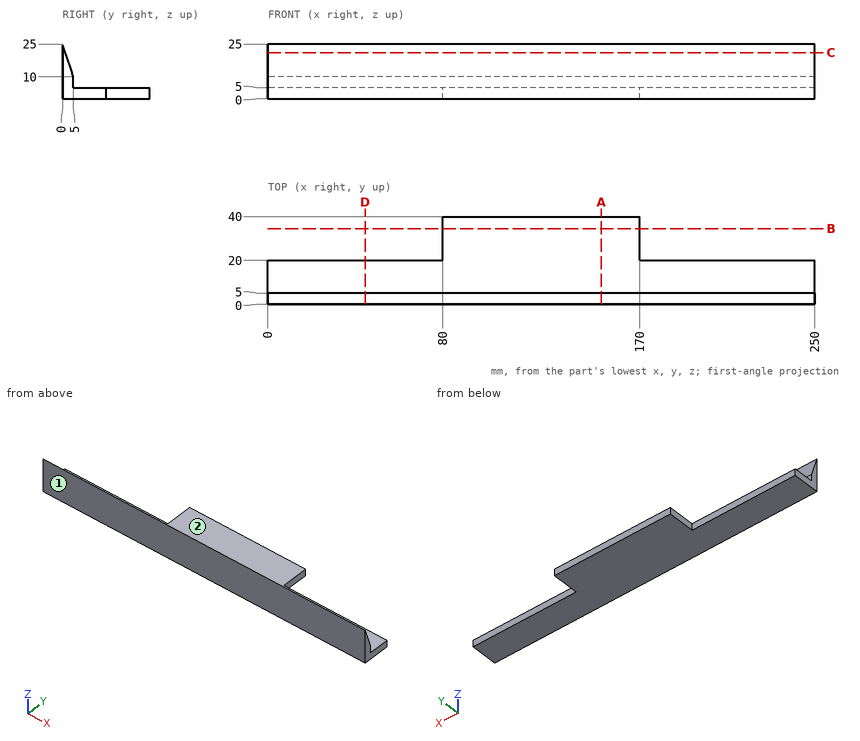
Answer from the drawing. Dimensions are ordinates in mm from the lowest x, y and z of the part. A direction names the side the tool comes from. Coordinates: 2 decimals unless noted, no trailing zeros. Write each loop counter-clockwise with the first axis right and the second up, starting at its lowest first coordinate (ties: lowest second). Pieces come first, ordered by that corner, then holes. Notation, with made-up numbers: (75.5, -25.75) - (129.5, -25.75) arc R22 ccw to (129.5, 11.25) - close; hole circle Ø4 at (87, 7.25). An arc over 180 degrees is marked (long way). Return JSON: item names as keys, results as strings. Group by question number.
Q1. Find the intervals of material crossed by line 1 along Z through (x, y) = (202, 9); line 2 along Y through (x, z) = (132, 21), in increasing order. Write a range as [from, to].
Q2. The part is cut by section C-C on z = 21. Write down the section's boundary in (x, y), and give its area (3 significant figures).
Q3. The part is cut by section D-D on x = 44.5. Write down the section's boundary in (y, z), and give its area (4 significant figures).
Q4. Flat-ended cylindrical pins translate along their axes: pin 1 Ø6 at (x, z) = (72.5, 4) entering from +Y; pin 2 Ø1.5 at (x, z) = (94, 8.5) entering from +Y; pin 3 Ø1.5 at (y, z) = (32, 2.5) entering from +X; pin 4 Ø6 at (x, y) = (126.5, 18.5) entering from -Z. Find the tip coordinate at first contact, or state that the pin passes through.
Q5. The part is cut by section B-B on y = 34.5. Write down the section's boundary in (x, z), and give its area (3 significant figures).
Q6. The part is cut by section A-A on x = 152.5. Write down the section's boundary in (y, z).
Q7. Which of the six approach directions +Z, -Z, +X, -X, +Y, -Y give full straight-line access (tool end or side, diameter ignored) to the marked faces 1 and 2?
Evaluation:
{
 "1": {"line 1": "z = [0, 5]", "line 2": "y = [0, 1.33]"},
 "2": {"outline": "(0, 0) - (250, 0) - (250, 1.33) - (0, 1.33) - close", "area": "333 mm2"},
 "3": {"outline": "(0, 0) - (20, 0) - (20, 5) - (5, 5) - (5, 10) - (0, 25) - close", "area": "162.5 mm2"},
 "4": {"pin 1": "stops at y = 20", "pin 2": "stops at y = 5", "pin 3": "stops at x = 170", "pin 4": "stops at z = 0"},
 "5": {"outline": "(80, 0) - (170, 0) - (170, 5) - (80, 5) - close", "area": "450 mm2"},
 "6": {"outline": "(0, 0) - (40, 0) - (40, 5) - (5, 5) - (5, 10) - (0, 25) - close"},
 "7": {"face 1": "+Z, -Z, +X, -X, -Y", "face 2": "+Z, +X, -X, +Y"}
}
